Could you check a few things on this model? Use its own coordinates, in mm. A direction names the side the tool comes from. Coordinates: 2 decimals unless noted, no trailing zeros. Order: outer loops, then holes, each group sorted by start corner. A loop starts at its lowest first (then second) coordinate and runs counter-clockwise, first axis right, second up. Notation, with made-up numbers: (29, 63.5) - (76, 63.5) arc R28 cw to (76, 100.5) - close; hole circle Ø10 at (1, 76). An arc over 180 degrees is marked (long way). Answer as CSV lines item,"result". Start each with the question number.
1. I want a section at D-D, the plane z = 25.5. List the corners of the cut face in (x, y) for me, and give its area (3 significant figures).
2. I want a section at B-B, the plane x = 139. List the corners of the cut face in (y, z) for me, and give its area (3 significant figures).
3. I want a section at A-A, the plane z = 14. List the corners of the cut face in (x, y) for me.
4. Thinking about a two-plate mould opening in Y: for faces 1 (the face through (145, -20, 14)), 2 (the face through (148, 78, 14)), 3 (the face through (143, 79, 14)), 4 (the face through (148, -7, 14)), which applies, released by +Y, released by -Y, zero draft, split by the parting line, or undercut?
5. For faces 5 (the face through (143, 29, 14)), 6 (the face through (143, -19, 14)), 7 (the face through (132.303, -12.423, 4.264)), which set-ups out of +Z, -Z, +X, -X, +Y, -Y let a thin tool reach every point of the face, with its end or its side?
6. For pin 1 (10 mm diameter, centred on x = 144.5, z = 22.5, fed in from -Y); pin 2 (9.5 mm diameter, centred on x = 143, z = 18.5, fed in from +Y); pin 3 (4 mm diameter, centred on y = 50, z = 11, fed in from -X); pin 4 (1.5 mm diameter, centred on x = 153.5, z = 20, fed in from +Y), each with a flat end and sliding along its axis, tell me the tip position at first contact or that it passes through.
7. I need wall thicknesses on probe 1 along Y at (x, z) = (148, 13.5); probe 2 along Z at (x, y) = (144.5, -12.5); probe 3 along X at (y, z) = (-11.5, 27). Which ranges of each line are inside material? Lowest first, please.
8. I want a section at C-C, the plane x = 145. List the corners of the cut face in (y, z) for me.
from build123d import *

# Parameters (mm, degrees)
CYLINDER002_R             = 16
CYLINDER002_DEPTH         = 11
CYLINDER002_ROLL_ANGLE    = 90
CYLINDER002001_R          = 16
CYLINDER002001_DEPTH      = 11
CYLINDER002001_ROLL_ANGLE = 90
CYLINDER_R                = 2
CYLINDER_DEPTH            = 100
CYLINDER_ROLL_ANGLE       = -90


with BuildPart() as wheel1:
    # Cylinder002 → Cylinder002 (new body)
    with BuildSketch(Plane.XY):
        Circle(CYLINDER002_R)
    extrude(amount=CYLINDER002_DEPTH)


with BuildPart() as wheel1_1:
    # Cylinder002 roll: moved
    add(wheel1.part.rotate(Axis((0, 0, 0), (1, 0, 0)), CYLINDER002_ROLL_ANGLE))


with BuildPart() as wheel1_2:
    # Cylinder002 placement: moved
    add(wheel1_1.part.moved(Location((20, -7, 14))))


with BuildPart() as wheel2:
    # Cylinder002001 → Cylinder002001 (new body)
    with BuildSketch(Plane.XY):
        Circle(CYLINDER002001_R)
    extrude(amount=CYLINDER002001_DEPTH)


with BuildPart() as wheel2_1:
    # Cylinder002001 roll: moved
    add(wheel2.part.rotate(Axis((0, 0, 0), (1, 0, 0)), CYLINDER002001_ROLL_ANGLE))


with BuildPart() as wheel2_2:
    # Cylinder002001 placement: moved
    add(wheel2_1.part.moved(Location((20, 78, 14))))


with BuildPart() as obj1:
    # Cylinder → Cylinder (new body)
    with BuildSketch(Plane.XY):
        Circle(CYLINDER_R)
    extrude(amount=CYLINDER_DEPTH)


with BuildPart() as obj1_1:
    # Cylinder roll: moved
    add(obj1.part.rotate(Axis((0, 0, 0), (1, 0, 0)), CYLINDER_ROLL_ANGLE))


with BuildPart() as obj1_2:
    # Cylinder placement: moved
    add(obj1_1.part.moved(Location((20, -20, 14))))

    # Fusion001: union Wheel1, Wheel2
    add(wheel1_2.part)
    add(wheel2_2.part)


with BuildPart() as obj1_3:
    # Fusion001 placement: moved
    add(obj1_2.part.moved(Location((125, 0, 0))))


solid = obj1_3.part
Solved:
1,outline,"(133.88, -18) - (156.12, -18) - (156.12, -7) - (133.88, -7) - close; (133.88, 67) - (156.12, 67) - (156.12, 78) - (133.88, 78) - close"
1,area,"489 mm2"
2,outline,"(-18, -0.83) - (-7, -0.83) - (-7, 28.83) - (-18, 28.83) - close; (67, -0.83) - (78, -0.83) - (78, 28.83) - (67, 28.83) - close"
2,area,"653 mm2"
3,outline,"(129, -18) - (143, -18) - (143, -20) - (147, -20) - (147, -18) - (161, -18) - (161, -7) - (147, -7) - (147, 67) - (161, 67) - (161, 78) - (147, 78) - (147, 80) - (143, 80) - (143, 78) - (129, 78) - (129, 67) - (143, 67) - (143, -7) - (129, -7) - close"
4,face 1,"released by -Y"
4,face 2,"released by +Y"
4,face 3,"zero draft"
4,face 4,"undercut"
5,face 5,"none"
5,face 6,"-Y"
5,face 7,"+Y, -Y"
6,pin 1,"stops at y = -18"
6,pin 2,"stops at y = 80"
6,pin 3,"stops at x = 143.27"
6,pin 4,"stops at y = 78"
7,probe 1,"y = -18 to -7, 67 to 78"
7,probe 2,"z = -1.99 to 29.99"
7,probe 3,"x = 135.67 to 154.33"
8,outline,"(-20, 12) - (-18, 12) - (-18, -2) - (-7, -2) - (-7, 12) - (67, 12) - (67, -2) - (78, -2) - (78, 12) - (80, 12) - (80, 16) - (78, 16) - (78, 30) - (67, 30) - (67, 16) - (-7, 16) - (-7, 30) - (-18, 30) - (-18, 16) - (-20, 16) - close"
